Verification items for the finished model (mm, model axes). Face numbers are marked on the shaded views. Coordinates: 2 decimals unless noted, no trailing zeros. Order: outer loops, then holes, each group sorted by start corner. A loop starts at its lowest first (then second) coordinate and runs counter-clockwise, first axis right, second up. Notation, with made-up numbers: M 62,-31.75 L 105,-31.75 A27 ccw 105,3.25 Z; hole C 41.5,71.25 d11. An arc over 180 degrees is marked long. Return JSON: item names as keys, results as strings. Group by question number.
1. Gauge pin test, flat ends, axial feed: pin 1 (1.5 mm diameter, centred on x = 4.5, z = 12.5, fed in from +Y); pin 2 (5 mm diameter, centred on y = -5, z = 4.5, fed in from -X); pin 3 (3 mm diameter, centred on x = 3.5, z = 15, fed in from +Y). Record the tip position at first contact, or that the pin passes through.
2. Section check C-C, the plane z = 14.75. Record the cut outline in (x, y), plus the area to 3 significant figures.
3. Material ranges on line 1 along Y through (x, z) = (0, 15.4); line 2 along Z through (x, y) = (1, 5); line 3 along Z through (x, y) = (3.75, 1), recorded low to high.
4. Mould release check, pull along X, two halves, no side actions. Record for the marked faces 1, 2 and 3: +X half, -X half, draft (parallel to the pull), parting line (faces both ways), or undercut.
5. Section check A-A, the plane x = 0. Record the cut outline in (y, z) (3 decimals), plus the area to 3 significant figures.
6. Section check D-D, the plane x = 3. Record the cut outline in (y, z), plus the area to 3 significant figures.
Autodesk Inventor part; units mm, degrees
ref_plane "YZ Plane" through (0, 0, 0) normal (1, 0, 0) x (0, 1, 0)
ref_plane "XZ Plane" through (0, 0, 0) normal (0, 1, 0) x (-1, 0, 0)
ref_plane "XY Plane" through (0, 0, 0) normal (0, 0, 1) x (1, 0, 0)
sketch "Sketch1" plane through (0, 0, 0) normal (0, 0, 1) x (1, 0, 0)
  circle A0 centre (0, 0) radius 7.5
  dimension "d0" = 15
extrude "Extrusion1" add sketch "Sketch1" along normal blind 16
sketch "Sketch2" plane through (0, 0, 16) normal (0, 0, 1) x (1, 0, 0)
  circle A0 centre (0, 0) radius 7.5
  circle A1 centre (0, 0) radius 1.2
  dimension "d3" = 2.4
extrude "Extrusion2" cut sketch "Sketch2" against normal blind 2 contours A1
sketch "Sketch3" plane through (0, 0, 16) normal (0, 0, 1) x (1, 0, 0)
  circle A0 centre (0, 0) radius 7.5
  circle A1 centre (0, 0) radius 1.9
  circle A2 centre (0, 0) radius 2.5
  dimension "d6" = 3.8
  dimension "d7" = 5
extrude "Extrusion3" add sketch "Sketch3" along normal blind 1 contours A2
sketch "Sketch4" plane through (0, 0, 16) normal (0, 0, 1) x (1, 0, 0)
  circle A0 centre (0, 0) radius 2.5
  circle A1 centre (0, 0) radius 5
  dimension "d10" = 10
extrude "Extrusion4" cut sketch "Sketch4" against normal blind 1
sketch "Sketch5" plane through (0, 0, 0) normal (0, 0, -1) x (-1, 0, 0)
  circle A0 centre (0, 0) radius 7.5
hole "Hole1" at (0, 0, 0) direction (0, 0, 1) diameter 1.05 end through all
sketch "Sketch6" plane through (0, 0, 17) normal (0, 0, 1) x (1, 0, 0)
  circle A0 centre (0, 0) radius 1.9
hole "Hole2" at (0, 0, 17) direction (0, 0, -1) diameter 4 depth 2.5
properties part number "Bearing_ID_Asm_Base"
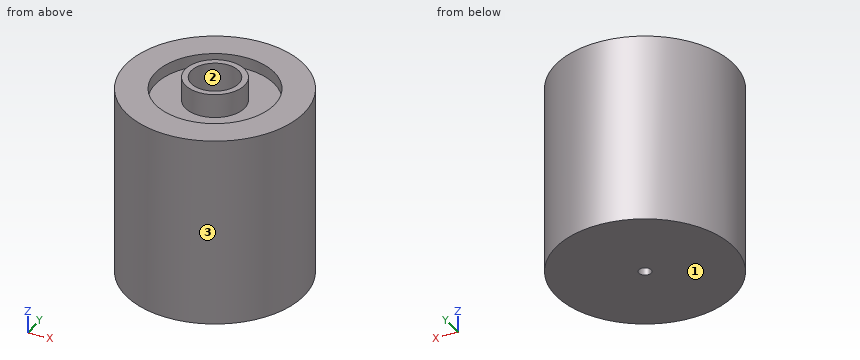
Answers follow:
{
 "1": {"pin 1": "y = 6.5", "pin 2": "x = -7.07", "pin 3": "y = 7.23"},
 "2": {"outline": "C 0,0 d15; hole C 0,0 d4", "area": "164 mm^2"},
 "3": {"line 1": "-7.5 to -5, -2.5 to -2, 2 to 2.5, 5 to 7.5", "line 2": "0 to 16", "line 3": "0 to 15"},
 "4": {"face 1": "draft", "face 2": "undercut", "face 3": "parting line"},
 "5": {"outline": "M -7.5,0 L -0.525,0 L -0.525,14 L -1.2,14 L -1.2,14.5 L -2,14.5 L -2,17 L -2.5,17 L -2.5,15 L -5,15 L -5,16 L -7.5,16 Z; M 0.525,0 L 7.5,0 L 7.5,16 L 5,16 L 5,15 L 2.5,15 L 2.5,17 L 2,17 L 2,14.5 L 1.2,14.5 L 1.2,14 L 0.525,14 Z", "area": "214 mm^2"},
 "6": {"outline": "M -6.87,0 L 6.87,0 L 6.87,16 L 4,16 L 4,15 L -4,15 L -4,16 L -6.87,16 Z", "area": "212 mm^2"}
}
